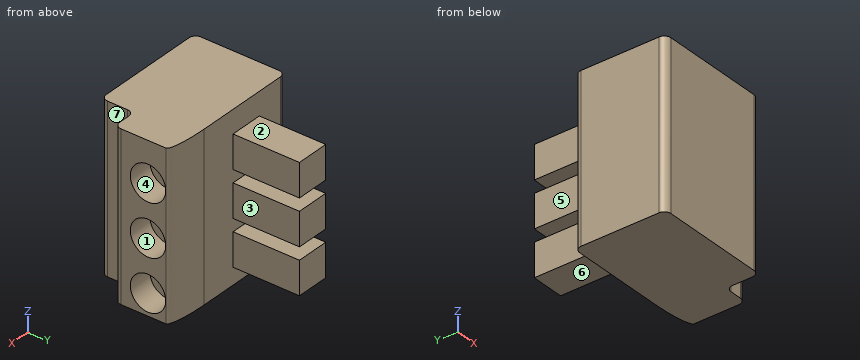
from build123d import *

# Parameters (mm, degrees)
SKETCH1_W           = 11.303
SKETCH1_H           = 15.6972
BOSS_EXTRUDE1_DEPTH = 8.73125
SKETCH2_W           = 15.6972
SKETCH2_H           = 5.55625
BOSS_EXTRUDE2_DEPTH = 2.38125
FILLET1_R           = 0.635
SKETCH5_R           = 1.69545
CUT_EXTRUDE1_DEPTH  = 2.38125
SKETCH7_W           = 3.175
SKETCH7_H           = 3.175
BOSS_EXTRUDE3_DEPTH = 6.35
FILLET2_SIZE        = 0.635
FILLET2_SIZE_2      = 3.81
FILLET3_R           = 0.635


with BuildPart() as part:
    # Sketch1 → Boss-Extrude1 (new body)
    with BuildSketch(Plane(origin=(0, 0, 0), x_dir=(1, 0, 0), z_dir=(0, 1, 0))):
        with Locations((5.6515, 7.8486)):
            Rectangle(SKETCH1_W, SKETCH1_H)
    extrude(amount=BOSS_EXTRUDE1_DEPTH)

    # Sketch2 → Boss-Extrude2 (add)
    with BuildSketch(Plane(origin=(11.303, 0, 0), x_dir=(0, 0, -1), z_dir=(1, 0, 0))):
        with Locations((7.8486, 5.953125)):
            Rectangle(SKETCH2_W, SKETCH2_H)
    extrude(amount=BOSS_EXTRUDE2_DEPTH)

    # Fillet1
    fillet1_edges = [part.edges().sort_by_distance(p)[0] for p in [
        (13.68425, 3.175, -7.8486),
    ]]
    fillet(fillet1_edges, radius=FILLET1_R)

    # Sketch5 → Cut-Extrude1 (cut)
    with BuildSketch(Plane(origin=(13.68425, 0, 0), x_dir=(0, 0, -1), z_dir=(1, 0, 0))):
        with Locations((13.64615, 6.39445)):
            Circle(SKETCH5_R)
        with Locations((8.73125, 6.39445)):
            Circle(SKETCH5_R)
        with Locations((3.81635, 6.39445)):
            Circle(SKETCH5_R)
    extrude(amount=-CUT_EXTRUDE1_DEPTH, mode=Mode.SUBTRACT)

    # Sketch7 → Boss-Extrude3 (add)
    with BuildSketch(Plane(origin=(0, 8.73125, 0), x_dir=(1, 0, 0), z_dir=(0, 1, 0))):
        with Locations((4.7625, 3.79095)):
            Rectangle(SKETCH7_W, SKETCH7_H)
        with Locations((4.7625, 12.5222)):
            Rectangle(SKETCH7_W, SKETCH7_H)
        with Locations((4.7625, 8.156575)):
            Rectangle(SKETCH7_W, SKETCH7_H)
    extrude(amount=BOSS_EXTRUDE3_DEPTH)

    # Fillet2
    # an asymmetric fillet: 3.81, 0.635 mm, written as the material it takes off along each edge
    with BuildSketch(Plane(origin=(13.68425, 8.73125, 9.525), x_dir=(0, -1, 0), z_dir=(0, 0, -1))) as fillet2_piece_1:
        with BuildLine():
            Bezier((FILLET2_SIZE, 0), (0, 0), (0, FILLET2_SIZE_2), weights=[1, 0.707106781, 1])
            Line((0, FILLET2_SIZE_2), (0, 0))
            Line((0, 0), (FILLET2_SIZE, 0))
        make_face()
    extrude(amount=34.7472, mode=Mode.SUBTRACT)

    # Fillet3
    fillet3_edges = [part.edges().sort_by_distance(p)[0] for p in [
        (11.303, 3.175, -7.8486),
        (11.303, 0, -7.8486),
        (0, 0, -7.8486),
        (0, 8.73125, -7.8486),
    ]]
    fillet(fillet3_edges, radius=FILLET3_R)


solid = part.part
Read the model definition and answer for the solid it produces. Units are mm, in the model's axes. Face numbers are marked on the shaded views. A direction names the side the tool comes from. Coordinates: 2 decimals unless noted, no trailing zeros. Order: outer loops, then holes, each group sorted by start corner. A loop starts at its lowest first (then second) coordinate and runs counter-clockwise, first axis right, second up. Notation, with made-up numbers: M -34.5,70 L -23.5,70 A37 cw -23.5,107 Z; hole C 60,4 d1. An arc over 180 degrees is marked long. Put each result on its own line as item: value. Start each with the question number.
Item 1: Section B-B, the plane x = 6 is taken. Determine the outline of the cut face in (y, z).
Item 2: Section A-A, the plane y = 10 is taken. Determine the outline of the cut face in (x, z) (3 decimals).
Item 3: Consider probe 1 along Z at (x, y) = (12, 6.25); probe 2 along Y at (x, z) = (10.25, -4.5); probe 3 along Y at (x, z) = (11.5, -13.5). Determine where each line is inside the solid, lowest interval first. Write a range as [from, to].
Item 4: The mould has two halves that part along Z. Classify the marked faces 1, 2 and 3: +Z half, -Z half, draft (parallel to the pull), parting line (faces both ways), or undercut.
Item 5: Section D-D, the plane x = 12.25 is taken. Count the separate pieces of the cut face and the enclosed holes in it, plus the area to 3 significant figures.
Item 6: For the marked faces 4, 5, 6 and 7, determine the directions among +Z, -Z, +X, -X, +Y, -Y from which every point of the face is accessible in a straight line to the end or side of a thin tool.
Item 7: Given pin 1 Ø0.6 at (y, z) = (1.5, -10.5) entering from +X; pin 2 Ø1.6 at (y, z) = (11, -4) entering from +X; pin 3 Ø1.6 at (y, z) = (10.5, -13) entering from -X (3 decimals), each flat-ended and moving along its own axis, determine where each tip first touches the part or whether it passes through.
Item 8: Section C-C, the plane y = 7.75 is taken. Determine the outline of the cut face in (x, z).
Computed:
1. outline: M 0,-15.7 L 8.73,-15.7 L 8.73,-14.11 L 15.08,-14.11 L 15.08,-10.93 L 8.73,-10.93 L 8.73,-9.74 L 15.08,-9.74 L 15.08,-6.57 L 8.73,-6.57 L 8.73,-5.38 L 15.08,-5.38 L 15.08,-2.2 L 8.73,-2.2 L 8.73,0 L 0,0 Z
2. outline: M 3.175,-14.11 L 6.35,-14.11 L 6.35,-10.935 L 3.175,-10.935 Z; M 3.175,-9.744 L 6.35,-9.744 L 6.35,-6.569 L 3.175,-6.569 Z; M 3.175,-5.378 L 6.35,-5.378 L 6.35,-2.203 L 3.175,-2.203 Z
3. probe 1: z = [-15.7, -15.34], [-11.96, -10.42], [-7.04, -5.51], [-2.13, 0]
3. probe 2: y = [0, 8.73]
3. probe 3: y = [3, 4.71], [8.08, 8.67]
4. face 1: undercut
4. face 2: +Z half
4. face 3: draft
5. separate pieces: 1
5. enclosed holes: 3
5. area: 58.0 mm2
6. face 4: +X
6. face 5: +Z, -Z, -X, +Y
6. face 6: -Z, +X, -X, +Y
6. face 7: +Z, -Z, +X, -Y
7. pin 1: stops at x = 11.3
7. pin 2: stops at x = 6.35
7. pin 3: stops at x = 3.175
8. outline: M 0,-15.7 L 13.68,-15.7 L 13.68,-14.66 L 11.3,-14.66 L 11.3,-12.63 L 13.68,-12.63 L 13.68,-9.75 L 11.3,-9.75 L 11.3,-7.71 L 13.68,-7.71 L 13.68,-4.83 L 11.3,-4.83 L 11.3,-2.8 L 13.68,-2.8 L 13.68,0 L 0,0 Z
